Geometry: final body of the model. Coordinates: model frame, mm. Face numbers are marked on the shaded views. A direction names the side the tool comes from. Round coordinates to 2 decimals unless told otherwise and drop trailing zeros. Loops run counter-clockwise (first coordinate to the right, second up) from the corner with the lowest first, then second, coordinate; pieces in that order, holes last. Notation, with made-up numbers: (80.5, 8.5) -> (123.5, 8.5) arc R17 cw to (123.5, 15.5) -> close; hole circle Ø6 at (60, 73). An arc over 180 degrees is marked (long way). Answer in a Markdown table with one row per item.
```python
from build123d import *

# Parameters (mm, degrees)
F0_W     = 860
F0_H     = 356
F1_DEPTH = 13
F2_W     = 13
F2_H     = 356
F3_DEPTH = 280
F4_W     = 834
F4_H     = 13
F5_DEPTH = 280
F7_DEPTH = 860


with BuildPart() as f1:
    # F0 (on Front) → F1 (new body)
    with BuildSketch(Plane.XZ):
        Rectangle(F0_W, F0_H)
    extrude(amount=F1_DEPTH)

    # F2 (on face) → F3 (join)
    with BuildSketch(Plane.XZ.offset(13)):
        with Locations((-423.5, 0)):
            Rectangle(F2_W, F2_H)
        with Locations((423.5, 0)):
            Rectangle(F2_W, F2_H)
    extrude(amount=F3_DEPTH)

    # F4 (on face) → F5 (join)
    with BuildSketch(Plane.XZ.offset(13)):
        with Locations((0, 171.5)):
            Rectangle(F4_W, F4_H)
        with Locations((0, -171.5)):
            Rectangle(F4_W, F4_H)
    extrude(amount=F5_DEPTH)

    # F6 (on face) → F7 (join, through all)
    with BuildSketch(Plane.YZ.offset(430)):
        Polygon((-270.6, 178), (-270.6, 181), (-296, 181), (-296, 155.6), (-293, 155.6), (-293, 178), align=None)
    extrude(amount=-F7_DEPTH)


solid = f1.part
```
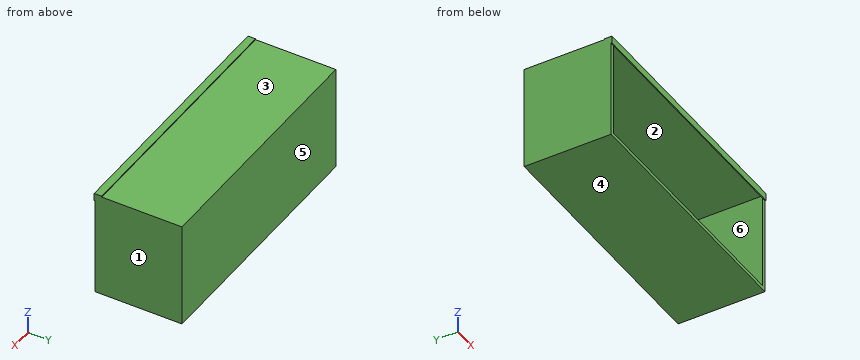
Item 1: Cut plane A-A (y = -207.5). Output: boundary loops of the cut face in (x, z), then the cut area to 3 significant figures.
Answer:
| item | result |
|---|---|
| outline | (-430, -178) -> (430, -178) -> (430, 178) -> (-430, 178) -> close; hole (-417, -165) -> (417, -165) -> (417, 165) -> (-417, 165) -> close |
| area | 30,900 mm² |
Item 2: Cut plane B-B (z = 147.5). Output: boundary loops of the cut face in (x, y).
Answer:
| item | result |
|---|---|
| outline | (-430, -293) -> (-417, -293) -> (-417, -13) -> (417, -13) -> (417, -293) -> (430, -293) -> (430, 0) -> (-430, 0) -> close |
Item 3: Draft query along Z for the marked faces 4, 5 and 6. Return one class per face: pulls with the +Z half, pulls with the -Z half, needs draft (parallel to the pull), parting line crosses it, or undercut.
Answer:
| item | result |
|---|---|
| face 4 | pulls with the -Z half |
| face 5 | needs draft |
| face 6 | undercut |
Item 4: Line query: probe 1 along Z at (x, y) = (162.5, -146.5); probe 2 along X at (y, z) = (-60, -63); probe 3 along Z at (x, y) = (305.5, -280). Output: solid intervals per line, ascending. Write a range as [from, to].
Answer:
| item | result |
|---|---|
| probe 1 | z = [-178, -165], [165, 178] |
| probe 2 | x = [-430, -417], [417, 430] |
| probe 3 | z = [-178, -165], [165, 181] |
Item 5: Pin query (flat end, axial travel): pin 1 Ø5 at (x, z) = (-291, -77) entering from -Y; pin 2 Ø12 at (x, y) = (65, -97.5) entering from +Z; pin 3 Ø1.5 at (x, y) = (-211, -295) entering from -Z. Return the tip coordinate at first contact, or that it passes through.
Answer:
| item | result |
|---|---|
| pin 1 | stops at y = -13 |
| pin 2 | stops at z = 178 |
| pin 3 | stops at z = 155.6 |
Item 6: Reachability of the marked faces 1, 2 and 3 from +Z, -Z, +X, -X, +Y, -Y: full face, straight path, thin tool, end or side. Return the list, or none.
Answer:
| item | result |
|---|---|
| face 1 | +Z, -Z, +X, +Y, -Y |
| face 2 | none |
| face 3 | +Z, +X, -X, +Y |
Item 7: Cut plane C-C (x = -139.5). Output: boundary loops of the cut face in (y, z), then the cut area to 3 significant figures.
Answer:
| item | result |
|---|---|
| outline | (-296, 155.6) -> (-293, 155.6) -> (-293, 165) -> (-13, 165) -> (-13, -165) -> (-293, -165) -> (-293, -178) -> (0, -178) -> (0, 178) -> (-270.6, 178) -> (-270.6, 181) -> (-296, 181) -> close |
| area | 12,100 mm² |
